Check sheet for the modelled part. Datum: model origin and axes. Units: mm. A direction names the side the tool comes from. Give positions to 0.01 mm unless a question says otherwise; leave off trailing zeros. Write each loop counter-clockwise with the first axis right and the second up, starting at its lowest first coordinate (ties: lowest second). Pieces come first, ordered by that corner, then holes. Notation, with made-up numbers: (-26.75, 13) -> (30.25, 13) arc R14 ccw to (30.25, 20) -> close; hole circle Ø10 at (10, 79.5). An arc over 180 degrees is marked (long way). Use a Markdown table: item, result. Add a question column.
1. Release check for a two-part mould opening along X. For faces 1 (the flat face through (-12.5, 9, 1)), 2 (the flat face through (0, 20, 2)), 3 (the cylindrical face through (-5.39, 1.01, 16.51)), 4 (the cylindrical face through (0.195, 1.014, 23.487)) record: released by +X, released by -X, zero draft, split by the parting line, or undercut.
2. Set-up check for faces 5 (the flat face through (0, 11.226, 1)), 6 (the flat face through (0, 0, 11)): record each of +Z, -Z, +X, -X, +Y, -Y from which the full face is reachable in a straight line by a thin tool's end or side.
3. Cross-section at C-C (x = 5.75). Enter the section's corners in (y, z), then the cut area to 3 significant figures.
4. Gauge pin test, flat ends, axial feed: P1, Ø4, axis at x = -7.5, z = 22, coming from the +Y side; P2, Ø2.5, axis at x = -6.5, z = 15.5, coming from the +Y side; P3, Ø2, axis at x = 9, y = 22.5, coming from the +Z side; P4, Ø6, axis at y = 27, z = 4, coming from the -X side. Record the tip position at first contact, or that the pin passes through.
5. Scan lines: probe 1 along Z at (x, y) = (0, 0.4); probe 2 along Z at (x, y) = (7.5, 17). Record each from-to range of solid material in increasing order. Write a range as [from, to].
6. Cross-section at A-A (z = 9). Enter the section's corners in (x, y), then the cut area to 3 significant figures.
7. Cross-section at D-D (z = 14.5). Enter the section's corners in (x, y).
from build123d import *

# Parameters (mm, degrees)
PAD_DEPTH       = 2
SKETCH001_W     = 25
SKETCH001_H     = 2
PAD001_DEPTH    = 26
SKETCH002_R     = 1.5
SKETCH002_R_2   = 4
POCKET_DEPTH    = 5
SKETCH003_R     = 1.5
SKETCH003_R_2   = 4
POCKET001_DEPTH = 5


with BuildPart() as part:
    # Sketch → Pad (new body)
    with BuildSketch(Plane.XY):
        with BuildLine():
            Line((-12.5, 0), (12.5, 0))
            Line((12.5, 0), (12.5, 24.5))
            ThreePointArc((12.5, 24.5), (0, 37), (-12.5, 24.5))
            Line((-12.5, 24.5), (-12.5, 0))
        make_face()
    extrude(amount=PAD_DEPTH)

    # Sketch001 (on Face6 of Pad) → Pad001 (join)
    with BuildSketch(Plane.XY.offset(2)):
        with Locations((0, 1)):
            Rectangle(SKETCH001_W, SKETCH001_H)
    extrude(amount=PAD001_DEPTH)

    # Sketch002 (on Face7 of Pad001) → Pocket (cut)
    with BuildSketch(Plane.XY.offset(2)):
        with Locations((0, 31)):
            Circle(SKETCH002_R)
        with Locations((0, 24.5)):
            Circle(SKETCH002_R_2)
        with Locations((0, 18)):
            Circle(SKETCH002_R)
        with Locations((6.5, 24.5)):
            Circle(SKETCH002_R)
        with Locations((-6.5, 24.5)):
            Circle(SKETCH002_R)
        Polygon((2.266718, 11.226343), (-2.266718, 11.226343), (0, 7.300272), align=None)
    extrude(amount=-POCKET_DEPTH, mode=Mode.SUBTRACT)

    # Sketch003 (on Face19 of Pocket) → Pocket001 (cut)
    with BuildSketch(Plane(origin=(0, 2, 0), x_dir=(-1, 0, 0), z_dir=(0, 1, 0))):
        with Locations((0, 22)):
            Circle(SKETCH003_R)
        with Locations((0, 15.5)):
            Circle(SKETCH003_R_2)
        with Locations((0, 9)):
            Circle(SKETCH003_R)
        with Locations((6.5, 15.5)):
            Circle(SKETCH003_R)
        with Locations((-6.5, 15.5)):
            Circle(SKETCH003_R)
        with BuildLine():
            ThreePointArc((12.5, 15.499975), (2.1e-05, 28), (-12.5, 15.500017))
            Line((-15.082001, 13.79535), (-12.5, 15.500017))
            Line((-17.874443, 34.459404), (-15.082001, 13.79535))
            Line((19.595028, 31.666967), (-17.874443, 34.459404))
            Line((12.5, 15.499975), (19.595028, 31.666967))
        make_face()
    extrude(amount=-POCKET001_DEPTH, mode=Mode.SUBTRACT)


solid = part.part
Worked answers:
| question | item | result |
|---|---|---|
| 1 | face 1 | released by -X |
| 1 | face 2 | zero draft |
| 1 | face 3 | undercut |
| 1 | face 4 | undercut |
| 2 | face 5 | +Z, -Z |
| 2 | face 6 | +Z, -Z, +X, -X, -Y |
| 3 | outline | (0, 0) -> (23.2, 0) -> (23.2, 2) -> (2, 2) -> (2, 14.2) -> (0, 14.2) -> close; (0, 16.8) -> (2, 16.8) -> (2, 26.6) -> (0, 26.6) -> close; (25.8, 0) -> (35.6, 0) -> (35.6, 2) -> (25.8, 2) -> close |
| 3 | area | 110 mm² |
| 4 | P1 | stops at y = 2 |
| 4 | P2 | passes through |
| 4 | P3 | stops at z = 2 |
| 4 | P4 | stops at x = -12.5 |
| 5 | probe 1 | z = [0, 7.5], [10.5, 11.5], [19.5, 20.5], [23.5, 28] |
| 5 | probe 2 | z = [0, 2] |
| 6 | outline | (-12.5, 0) -> (-1.5, 0) -> (-1.5, 2) -> (-12.5, 2) -> close; (1.5, 0) -> (12.5, 0) -> (12.5, 2) -> (1.5, 2) -> close |
| 6 | area | 44.0 mm² |
| 7 | outline | (-12.5, 0) -> (-7.62, 0) -> (-7.62, 2) -> (-12.5, 2) -> close; (-5.38, 0) -> (-3.87, 0) -> (-3.87, 2) -> (-5.38, 2) -> close; (3.87, 0) -> (5.38, 0) -> (5.38, 2) -> (3.87, 2) -> close; (7.62, 0) -> (12.5, 0) -> (12.5, 2) -> (7.62, 2) -> close |
